Can you work these out from the model? Positions are in its coordinate system, mm. Face numbers are marked on the shaded views. A direction names the side the tool comes from. Coordinates: 2 decimals unless noted, no trailing zeros. Order: outer loops, then holes, each group sorted by start corner. A loop starts at its lowest first (then second) coordinate and runs counter-clockwise, first axis right, second up. Notation, with made-up numbers: (45.25, 58.5) - (63.25, 58.5) arc R28 cw to (63.25, 88.5) - close; hole circle Ø9 at (-13.5, 1). An arc over 180 degrees is marked (long way). Return JSON: item names as keys, results as strings. Group by question number.
1) Imagine slicing it at B-B (y = -39). Write out the boundary of the cut face in (x, z), and give its area (3 significant figures).
2) For pin 1 Ø5 at (y, z) = (44.5, -1) entering from +X; pin 2 Ø9 at (x, y) = (6.5, -71) entering from +Z; pin 3 Ø4 at (x, z) = (-9.5, 5.5) entering from +Y, each with a flat end and sliding along its axis, tell me the tip position at first contact or that it passes through.
3) Imagine slicing it at D-D (y = 33). Write out the boundary of the cut face in (x, z).
4) Imagine slicing it at A-A (x = 0). Write out the boundary of the cut face in (y, z).
5) Imagine slicing it at C-C (z = -3). Write out the boundary of the cut face in (x, y).
6) If we mould it in two halves opening along X, with no side actions, what happens to the marked faces 1, 2, 3 and 4? For each: pulls with the +X half, pulls with the -X half, needs draft (parallel to the pull), parting line crosses it, or undercut.
7) Which directions (+Z, -Z, +X, -X, +Y, -Y) give clear straight access to the entire face, cutting with the end or side of a thin tool? Please do the marked faces 5, 6, 7 and 8.
8) If I drill on line 1 along Y through (x, z) = (0, -6); line 2 along Y through (x, z) = (0, -4); line 3 along Y through (x, z) = (7.5, 6.5), over which ranges is the centre line in solid material (lowest first)?
```python
from build123d import *

# Parameters (mm, degrees)
SKETCH2_R             = 21
SKETCH2_R_2           = 16
BOSS_EXTRUDE1_DEPTH   = 10
SKETCH2_R_3           = 12.5
SKETCH2_R_4           = 6.25
BOSS_EXTRUDE1_2_DEPTH = 10
BOSS_EXTRUDE2_DEPTH   = 5


with BuildPart() as part:
    # Sketch2 → Boss-Extrude1 (new, symmetric)
    with BuildSketch(Plane.XY):
        with Locations((0, -43.810288723)):
            Circle(SKETCH2_R)
        with Locations((0, -43.810288723)):
            Circle(SKETCH2_R_2, mode=Mode.SUBTRACT)
    extrude(amount=BOSS_EXTRUDE1_DEPTH, both=True)



with BuildPart() as body_2:
    # Sketch2 → Boss-Extrude1 2 (new, symmetric)
    with BuildSketch(Plane.XY):
        with Locations((0, 76.189711277)):
            Circle(SKETCH2_R_3)
        with Locations((0, 76.189711277)):
            Circle(SKETCH2_R_4, mode=Mode.SUBTRACT)
    extrude(amount=BOSS_EXTRUDE1_2_DEPTH, both=True)


with BuildPart() as part_1:
    add(part.part)

    add(body_2.part)  # Boss-Extrude2 merges body 2
    # Sketch2<3> → Boss-Extrude2 (add, symmetric)
    with BuildSketch(Plane.XY):
        with BuildLine():
            ThreePointArc((-8.40143978, 21.934128658), (-11.204201439, -7.583899174), (-19.512314514, -36.046940071))
            ThreePointArc((-19.512314514, -36.046940071), (0, -22.810288723), (19.512314514, -36.046940071))
            ThreePointArc((19.512314514, -36.046940071), (11.204201439, -7.583899174), (8.40143978, 21.934128658))
            Line((8.40143978, 21.934128658), (8.40143978, 66.934128658))
            ThreePointArc((8.40143978, 66.934128658), (0, 63.689711277), (-8.40143978, 66.934128658))
            Line((-8.40143978, 66.934128658), (-8.40143978, 21.934128658))
        make_face()
        with BuildLine():
            Line((-6.10309837, 93.714824033), (-6.10309837, 87.098523783))
            ThreePointArc((-6.10309837, 87.098523783), (0.131172403, 88.68902301), (6.330691245, 86.968038993))
            Line((6.330691245, 86.968038993), (6.330691245, 93.714824033))
            Line((6.330691245, 93.714824033), (-6.10309837, 93.714824033))
        make_face()
        with BuildLine():
            ThreePointArc((14.185268549, -59.295060475), (1.002030285, -64.786368798), (-12.644623669, -60.576728186))
            Line((-12.644623669, -60.576728186), (-12.644623669, -76.805395819))
            Line((-12.644623669, -76.805395819), (14.185268549, -76.805395819))
            Line((14.185268549, -76.805395819), (14.185268549, -59.295060475))
        make_face()
    extrude(amount=BOSS_EXTRUDE2_DEPTH, both=True)


solid = part_1.part
```
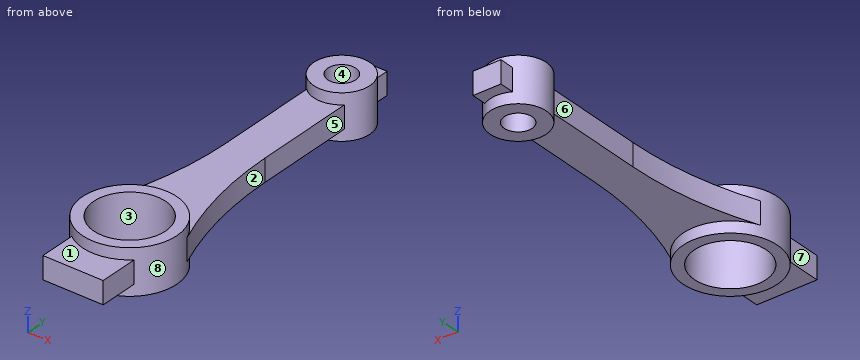
Calculated:
{
 "1": {"outline": "(-20.44, -10) - (-15.26, -10) - (-15.26, 10) - (-20.44, 10) - close; (15.26, -10) - (20.44, -10) - (20.44, 10) - (15.26, 10) - close", "area": "207 mm2"},
 "2": {"pin 1": "x = 8.4", "pin 2": "z = 5", "pin 3": "y = 86.19"},
 "3": {"outline": "(-8.4, -5) - (8.4, -5) - (8.4, 5) - (-8.4, 5) - close"},
 "4": {"outline": "(-76.81, -5) - (-64.81, -5) - (-64.81, -10) - (-59.81, -10) - (-59.81, 10) - (-64.81, 10) - (-64.81, 5) - (-76.81, 5) - close; (-27.81, -10) - (-22.81, -10) - (-22.81, -5) - (63.69, -5) - (63.69, -10) - (69.94, -10) - (69.94, 10) - (63.69, 10) - (63.69, 5) - (-22.81, 5) - (-22.81, 10) - (-27.81, 10) - close; (82.44, -10) - (88.69, -10) - (88.69, -5) - (93.71, -5) - (93.71, 5) - (88.69, 5) - (88.69, 10) - (82.44, 10) - close"},
 "5": {"outline": "(-19.51, -36.05) arc R21 ccw to (-12.64, -60.58) - (-12.64, -76.81) - (14.19, -76.81) - (14.19, -59.3) arc R21 ccw to (19.51, -36.05) arc R156.84 cw to (8.4, 21.93) - (8.4, 66.93) arc R12.5 ccw to (6.33, 86.97) - (6.33, 93.71) - (-6.1, 93.71) - (-6.1, 87.1) arc R12.5 ccw to (-8.4, 66.93) - (-8.4, 21.93) arc R156.84 cw to start; hole circle Ø32 at (0, -43.81); hole circle Ø12.5 at (0, 76.19)"},
 "6": {"face 1": "needs draft", "face 2": "pulls with the +X half", "face 3": "undercut", "face 4": "undercut"},
 "7": {"face 5": "+Z, -Z, +X", "face 6": "+Z, -Z, -X", "face 7": "+Z, -Z, -X, -Y", "face 8": "none"},
 "8": {"line 1": "-64.81 to -59.81, -27.81 to -22.81, 63.69 to 69.94, 82.44 to 88.69", "line 2": "-76.81 to -59.81, -27.81 to 69.94, 82.44 to 93.71", "line 3": "-63.43 to -57.94, -29.68 to -24.2, 66.19 to 86.19"}
}
